Part print with two shaded views. Sizes in mm from the minimum x, y, z corner. A direction names the side the tool comes from. Give positions to 0.01 mm unless a question says otherwise; leave off trailing zeros. Write each loop counter-clockwise with the first axis right and the second up, starting at its lowest first coordinate (ties: lowest second). Pieces come first, ordered by that corner, then holes.
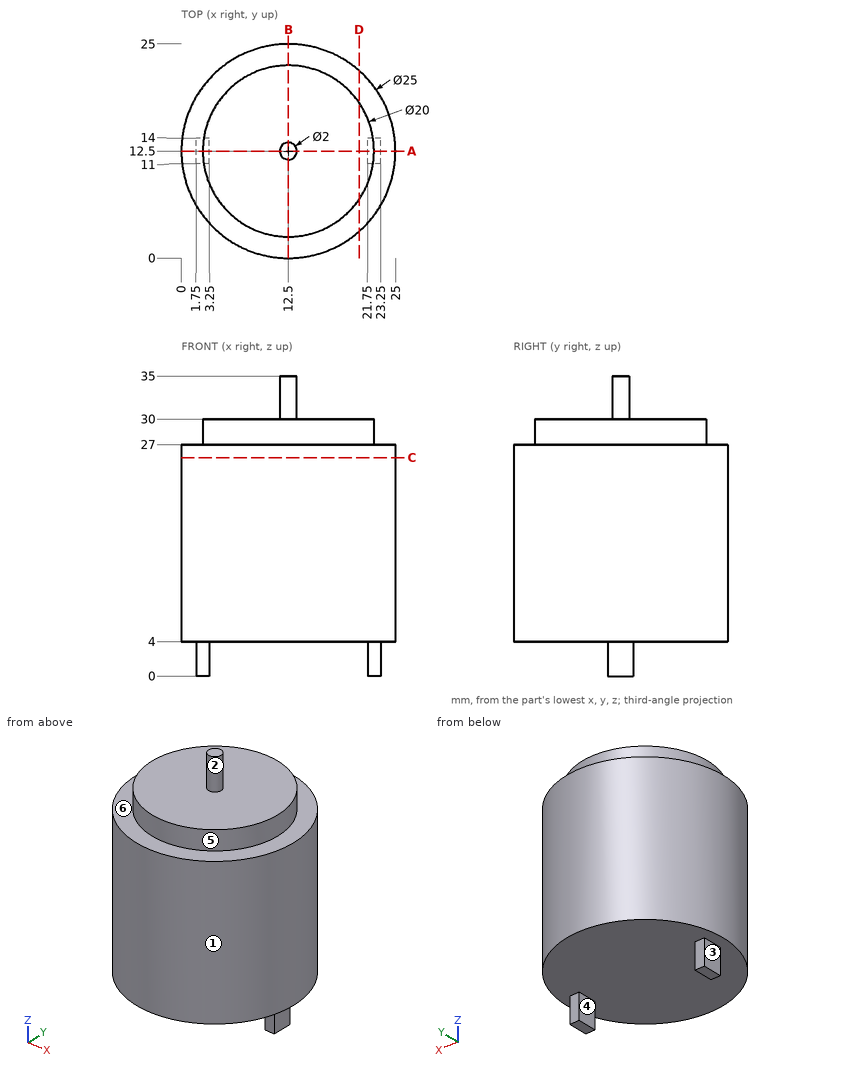
1) Saw through at A-A (y = 12.5). Write the cut outline in (x, z), and give its area (3 significant figures).
Check result:
outline: (0, 4) - (1.75, 4) - (1.75, 0) - (3.25, 0) - (3.25, 4) - (21.75, 4) - (21.75, 0) - (23.25, 0) - (23.25, 4) - (25, 4) - (25, 27) - (22.5, 27) - (22.5, 30) - (13.5, 30) - (13.5, 35) - (11.5, 35) - (11.5, 30) - (2.5, 30) - (2.5, 27) - (0, 27) - close
area: 657 mm2
2) 3-axis set-ups, long thin cutter, end or side, ignore diameter. For the marked faces 1 and 2: which of +Z, -Z, +X, -X, +Y, -Y reach the whole face in a straight line?
Check result:
face 1: +Z, -Z
face 2: +Z
3) Drill centre lines: L1, parallel to Z at x = 21, y = 15.25; L2, parallel to X at y = 12.25, z = 20.5; L3, parallel to Y at x = 12, z = 17. Where is each one in solid material? Low to high.
Check result:
L1: z = 4 to 30
L2: x = 0 to 25
L3: y = 0.01 to 24.99
4) Mould opens along X. For the marked faces 3, 4, 5 and 6 say: +X half, -X half, draft (parallel to the pull), parting line (faces both ways), or undercut.
Check result:
face 3: -X half
face 4: undercut
face 5: parting line
face 6: draft
5) Saw through at C-C (z = 25.5). Write the cut outline in (x, y).
Check result:
outline: circle Ø25 at (12.5, 12.5)
6) Flat gauge pins, fed straight in: P1, Ø2.5, axis at y = 13, z = 1.5, coming from the +X side; P2, Ø5, axis at x = 5.5, y = 22, coming from the -Z side; P3, Ø1, axis at x = 7.5, z = 30, coming from the -Y side. Where does each tip first touch, or does it go through?
Check result:
P1: stops at x = 23.25
P2: stops at z = 4
P3: stops at y = 3.57
7) Saw through at D-D (x = 20.75). Write the cut outline in (y, z).
Check result:
outline: (3.11, 4) - (21.89, 4) - (21.89, 27) - (18.15, 27) - (18.15, 30) - (6.85, 30) - (6.85, 27) - (3.11, 27) - close
8) Saw through at B-B (x = 12.5). Write the cut outline in (y, z).
Check result:
outline: (0, 4) - (25, 4) - (25, 27) - (22.5, 27) - (22.5, 30) - (13.5, 30) - (13.5, 35) - (11.5, 35) - (11.5, 30) - (2.5, 30) - (2.5, 27) - (0, 27) - close
